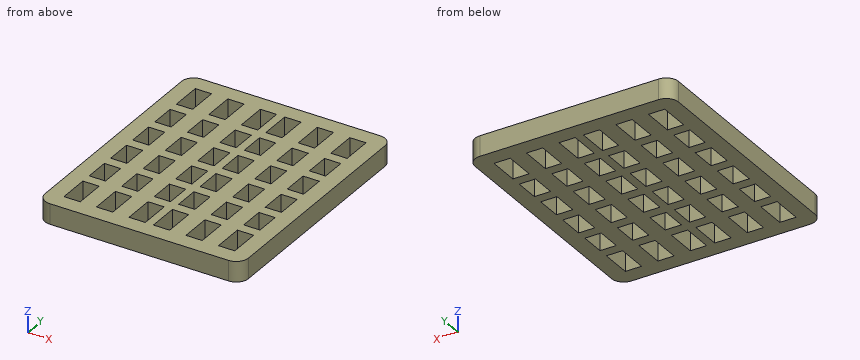
from build123d import *

# Parameters (mm, degrees)
F1_DEPTH = 5
F0_W     = 4
F0_H     = 7.5
F0_H_2   = 6.25
F0_H_3   = 6
F0_W_2   = 2
F0_H_4   = 2.5
F2_DEPTH = 5


# Not quite as in the source:
# - a feature names something its author has since deleted; it is built from what else it names


with BuildPart() as f1:
    # F0 (on Top) → F1 (new body)
    with BuildSketch(Plane.XY):
        with BuildLine():
            ThreePointArc((0, 3), (0.8786796564, 0.8786796564), (3, 0))
            Line((3, 0), (47, 0))
            ThreePointArc((47, 0), (49.1213203436, 0.8786796564), (50, 3))
            Line((50, 3), (50, 57))
            ThreePointArc((50, 57), (49.1213203436, 59.1213203436), (47, 60))
            Line((47, 60), (25, 60))
            Line((25, 60), (3, 60))
            ThreePointArc((3, 60), (0.8786796564, 59.1213203436), (0, 57))
            Line((0, 57), (0, 3))
        make_face()
        Polygon((24, 56), (25, 56), (26, 56), (30, 56), (34, 56), (38, 56), (42, 56), (46, 56), (46, 48.5), (46, 46), (46, 40), (46, 37.5), (46, 31.25), (46, 28.75), (46, 22.5), (46, 20), (46, 14), (46, 11.5), (46, 4), (42, 4), (38, 4), (34, 4), (30, 4), (26, 4), (24, 4), (20, 4), (16, 4), (12, 4), (8, 4), (4, 4), (4, 11.5), (4, 14), (4, 20), (4, 22.5), (4, 28.75), (4, 31.25), (4, 37.5), (4, 40), (4, 46), (4, 48.5), (4, 56), (8, 56), (12, 56), (16, 56), (20, 56), align=None, mode=Mode.SUBTRACT)
    extrude(amount=F1_DEPTH)

    # F0 (on Top) → F2 (join)
    with BuildSketch(Plane.XY):
        with BuildLine():
            ThreePointArc((0, 3), (0.8786796564, 0.8786796564), (3, 0))
            Line((3, 0), (47, 0))
            ThreePointArc((47, 0), (49.1213203436, 0.8786796564), (50, 3))
            Line((50, 3), (50, 57))
            ThreePointArc((50, 57), (49.1213203436, 59.1213203436), (47, 60))
            Line((47, 60), (25, 60))
            Line((25, 60), (3, 60))
            ThreePointArc((3, 60), (0.8786796564, 59.1213203436), (0, 57))
            Line((0, 57), (0, 3))
        make_face()
        Polygon((24, 56), (25, 56), (26, 56), (30, 56), (34, 56), (38, 56), (42, 56), (46, 56), (46, 48.5), (46, 46), (46, 40), (46, 37.5), (46, 31.25), (46, 28.75), (46, 22.5), (46, 20), (46, 14), (46, 11.5), (46, 4), (42, 4), (38, 4), (34, 4), (30, 4), (26, 4), (24, 4), (20, 4), (16, 4), (12, 4), (8, 4), (4, 4), (4, 11.5), (4, 14), (4, 20), (4, 22.5), (4, 28.75), (4, 31.25), (4, 37.5), (4, 40), (4, 46), (4, 48.5), (4, 56), (8, 56), (12, 56), (16, 56), (20, 56), align=None, mode=Mode.SUBTRACT)
        with Locations((18, 52.25)):
            Rectangle(F0_W, F0_H)
        with Locations((32, 52.25)):
            Rectangle(F0_W, F0_H)
        with Locations((10, 52.25)):
            Rectangle(F0_W, F0_H)
        with Locations((40, 52.25)):
            Rectangle(F0_W, F0_H)
        with Locations((18, 7.75)):
            Rectangle(F0_W, F0_H)
        with Locations((32, 7.75)):
            Rectangle(F0_W, F0_H)
        with Locations((10, 7.75)):
            Rectangle(F0_W, F0_H)
        with Locations((40, 7.75)):
            Rectangle(F0_W, F0_H)
        with Locations((18, 34.375)):
            Rectangle(F0_W, F0_H_2)
        with Locations((32, 34.375)):
            Rectangle(F0_W, F0_H_2)
        with Locations((10, 34.375)):
            Rectangle(F0_W, F0_H_2)
        with Locations((18, 25.625)):
            Rectangle(F0_W, F0_H_2)
        with Locations((40, 34.375)):
            Rectangle(F0_W, F0_H_2)
        with Locations((32, 25.625)):
            Rectangle(F0_W, F0_H_2)
        with Locations((10, 25.625)):
            Rectangle(F0_W, F0_H_2)
        with Locations((40, 25.625)):
            Rectangle(F0_W, F0_H_2)
        with Locations((18, 43)):
            Rectangle(F0_W, F0_H_3)
        with Locations((32, 43)):
            Rectangle(F0_W, F0_H_3)
        with Locations((10, 43)):
            Rectangle(F0_W, F0_H_3)
        with Locations((40, 43)):
            Rectangle(F0_W, F0_H_3)
        with Locations((18, 17)):
            Rectangle(F0_W, F0_H_3)
        with Locations((32, 17)):
            Rectangle(F0_W, F0_H_3)
        with Locations((10, 17)):
            Rectangle(F0_W, F0_H_3)
        with Locations((40, 17)):
            Rectangle(F0_W, F0_H_3)
        Polygon((26, 56), (25, 56), (24, 56), (24, 48.5), (26, 48.5), align=None)
        with Locations((25, 7.75)):
            Rectangle(F0_W_2, F0_H)
        with Locations((25, 34.375)):
            Rectangle(F0_W_2, F0_H_2)
        with Locations((25, 25.625)):
            Rectangle(F0_W_2, F0_H_2)
        with Locations((25, 43)):
            Rectangle(F0_W_2, F0_H_3)
        with Locations((25, 17)):
            Rectangle(F0_W_2, F0_H_3)
        with Locations((22, 47.25)):
            Rectangle(F0_W, F0_H_4)
        with Locations((28, 47.25)):
            Rectangle(F0_W, F0_H_4)
        with Locations((18, 47.25)):
            Rectangle(F0_W, F0_H_4)
        with Locations((32, 47.25)):
            Rectangle(F0_W, F0_H_4)
        with Locations((14, 47.25)):
            Rectangle(F0_W, F0_H_4)
        with Locations((22, 38.75)):
            Rectangle(F0_W, F0_H_4)
        with Locations((36, 47.25)):
            Rectangle(F0_W, F0_H_4)
        with Locations((28, 38.75)):
            Rectangle(F0_W, F0_H_4)
        with Locations((10, 47.25)):
            Rectangle(F0_W, F0_H_4)
        with Locations((18, 38.75)):
            Rectangle(F0_W, F0_H_4)
        with Locations((40, 47.25)):
            Rectangle(F0_W, F0_H_4)
        with Locations((32, 38.75)):
            Rectangle(F0_W, F0_H_4)
        with Locations((6, 47.25)):
            Rectangle(F0_W, F0_H_4)
        with Locations((14, 38.75)):
            Rectangle(F0_W, F0_H_4)
        with Locations((22, 30)):
            Rectangle(F0_W, F0_H_4)
        with Locations((44, 47.25)):
            Rectangle(F0_W, F0_H_4)
        with Locations((36, 38.75)):
            Rectangle(F0_W, F0_H_4)
        with Locations((28, 30)):
            Rectangle(F0_W, F0_H_4)
        with Locations((10, 38.75)):
            Rectangle(F0_W, F0_H_4)
        with Locations((18, 30)):
            Rectangle(F0_W, F0_H_4)
        with Locations((40, 38.75)):
            Rectangle(F0_W, F0_H_4)
        with Locations((32, 30)):
            Rectangle(F0_W, F0_H_4)
        with Locations((6, 38.75)):
            Rectangle(F0_W, F0_H_4)
        with Locations((14, 30)):
            Rectangle(F0_W, F0_H_4)
        with Locations((22, 21.25)):
            Rectangle(F0_W, F0_H_4)
        with Locations((44, 38.75)):
            Rectangle(F0_W, F0_H_4)
        with Locations((36, 30)):
            Rectangle(F0_W, F0_H_4)
        with Locations((28, 21.25)):
            Rectangle(F0_W, F0_H_4)
        with Locations((10, 30)):
            Rectangle(F0_W, F0_H_4)
        with Locations((18, 21.25)):
            Rectangle(F0_W, F0_H_4)
        with Locations((40, 30)):
            Rectangle(F0_W, F0_H_4)
        with Locations((32, 21.25)):
            Rectangle(F0_W, F0_H_4)
        with Locations((6, 30)):
            Rectangle(F0_W, F0_H_4)
        with Locations((14, 21.25)):
            Rectangle(F0_W, F0_H_4)
        with Locations((22, 12.75)):
            Rectangle(F0_W, F0_H_4)
        with Locations((44, 30)):
            Rectangle(F0_W, F0_H_4)
        with Locations((36, 21.25)):
            Rectangle(F0_W, F0_H_4)
        with Locations((28, 12.75)):
            Rectangle(F0_W, F0_H_4)
        with Locations((10, 21.25)):
            Rectangle(F0_W, F0_H_4)
        with Locations((18, 12.75)):
            Rectangle(F0_W, F0_H_4)
        with Locations((40, 21.25)):
            Rectangle(F0_W, F0_H_4)
        with Locations((32, 12.75)):
            Rectangle(F0_W, F0_H_4)
        with Locations((6, 21.25)):
            Rectangle(F0_W, F0_H_4)
        with Locations((14, 12.75)):
            Rectangle(F0_W, F0_H_4)
        with Locations((44, 21.25)):
            Rectangle(F0_W, F0_H_4)
        with Locations((36, 12.75)):
            Rectangle(F0_W, F0_H_4)
        with Locations((10, 12.75)):
            Rectangle(F0_W, F0_H_4)
        with Locations((40, 12.75)):
            Rectangle(F0_W, F0_H_4)
        with Locations((6, 12.75)):
            Rectangle(F0_W, F0_H_4)
        with Locations((44, 12.75)):
            Rectangle(F0_W, F0_H_4)
        with Locations((25, 47.25)):
            Rectangle(F0_W_2, F0_H_4)
        with Locations((25, 38.75)):
            Rectangle(F0_W_2, F0_H_4)
        with Locations((25, 30)):
            Rectangle(F0_W_2, F0_H_4)
        with Locations((25, 21.25)):
            Rectangle(F0_W_2, F0_H_4)
        with Locations((25, 12.75)):
            Rectangle(F0_W_2, F0_H_4)
    extrude(amount=F2_DEPTH)


solid = f1.part
Check sheet for the modelled part. Datum: model origin and axes. Units: mm. Give positions to 0.01 mm unless a question says otherwise; leave off trailing zeros. Write each loop counter-clockwise with the first axis right and the second up, starting at its lowest first coordinate (ties: lowest second). Pieces come first, ordered by that corner, then holes. Notation, with made-up numbers: (-18, -4.5) -> (40, -4.5) arc R10 cw to (40, 1.5) -> close; hole circle Ø4 at (-24, -8). An arc over 180 degrees is marked (long way). One line per item, written item: value. Start each with the question number.
Item 1: Section check C-C on z = 2.25. State how many separate pieces and enclosed holes the cut face has, then the cut area to 3 significant figures.
Item 2: Section check B-B on x = 36. Record the cut outline in (y, z).
Item 3: Section check A-A on y = 25. Record the cut outline in (x, z).
Item 4: Material ranges on probe 1 along Y at (x, z) = (2.5, 3.3), recorded low to high. Write a range as from..to.
Results list:
1. separate pieces: 1
1. enclosed holes: 36
1. area: 2,040 mm²
2. outline: (0, 0) -> (4, 0) -> (4, 5) -> (0, 5) -> close; (11.5, 0) -> (14, 0) -> (14, 5) -> (11.5, 5) -> close; (20, 0) -> (22.5, 0) -> (22.5, 5) -> (20, 5) -> close; (28.75, 0) -> (31.25, 0) -> (31.25, 5) -> (28.75, 5) -> close; (37.5, 0) -> (40, 0) -> (40, 5) -> (37.5, 5) -> close; (46, 0) -> (48.5, 0) -> (48.5, 5) -> (46, 5) -> close; (56, 0) -> (60, 0) -> (60, 5) -> (56, 5) -> close
3. outline: (0, 0) -> (4, 0) -> (4, 5) -> (0, 5) -> close; (8, 0) -> (12, 0) -> (12, 5) -> (8, 5) -> close; (16, 0) -> (20, 0) -> (20, 5) -> (16, 5) -> close; (24, 0) -> (26, 0) -> (26, 5) -> (24, 5) -> close; (30, 0) -> (34, 0) -> (34, 5) -> (30, 5) -> close; (38, 0) -> (42, 0) -> (42, 5) -> (38, 5) -> close; (46, 0) -> (50, 0) -> (50, 5) -> (46, 5) -> close
4. probe 1: 0.04..59.96
